```python
from build123d import *

# Parameters (mm, degrees)
RESSALTO_EXTRUS_O1_DEPTH = 1.5
ESBO_O2_R                = 0.1
RESSALTO_EXTRUS_O2_DEPTH = 0.1


with BuildPart() as part:
    # Esboço1 → Ressalto-extrusão1 (new body)
    with BuildSketch(Plane(origin=(0, 0, 0), x_dir=(1, 0, 0), z_dir=(0, 1, 0))):
        with BuildLine():
            Line((-3.97649343, 1.5), (-15, 1.5))
            ThreePointArc((-15, 1.5), (-16.358835062, 2.062847912), (-16.921682974, 3.421682974))
            Line((-16.921682974, 3.421682974), (-16.921682974, -3))
            ThreePointArc((-16.921682974, -3), (-16.482343146, -1.939339828), (-15.421682974, -1.5))
            Line((-15.421682974, -1.5), (-3.97649343, -1.5))
            ThreePointArc((-3.97649343, -1.5), (4.25, 0), (-3.97649343, 1.5))
        make_face()
    extrude(amount=RESSALTO_EXTRUS_O1_DEPTH)

    # Esboço2 → Ressalto-extrusão2 (add)
    with BuildSketch(Plane(origin=(0, 1.5, 0), x_dir=(1, 0, 0), z_dir=(0, 1, 0))):
        Circle(ESBO_O2_R)
    extrude(amount=RESSALTO_EXTRUS_O2_DEPTH)


solid = part.part
```
Build history of the part. All positions in model axes, mm. A direction names the side the tool comes from. Coordinates: 2 decimals unless noted, no trailing zeros. Order: outer loops, then holes, each group sorted by start corner. A loop starts at its lowest first (then second) coordinate and runs counter-clockwise, first axis right, second up. Notation, with made-up numbers: M 33,4 L 74,4 A20 ccw 74,38 Z; hole C -37.75,89 d2. An arc over 180 degrees is marked long. One line per question, with ' | ' between items. Start each with the question number.
1. Tool access for faces 4 (the face through (-16.494, 0.74, 1.951)), 5 (the face through (-9, 1, -1.5)), 6 (the face through (4.247, 0.74, 0.165)): list every direction of +Z, -Z, +X, -X, +Y, -Y with a clear straight run to the whole face (end or side of a thin tool).
2. Cut at C-C (x = -8.5). Write the cut outline in (y, z), plus the area to 3 significant figures.
3. Cut at B-B (z = 2.25). Write the cut outline in (x, y).
4. Cut at A-A (y = 0.85). Write the cut outline in (x, z).
5. Mould opens along X. For faces 1 (the face through (-4, 1.5, 0)), 2 (the face through (-16.344, 0.74, -2.048)), 3 (the face through (-16.922, 1, 0)) say: +X half, -X half, draft (parallel to the pull), parting line (faces both ways), or undercut.
6. Cut at D-D (z = 3.5). Write the cut outline in (x, y).
7. Flat gauge pins, fed straight in: P1, Ø0.8, axis at x = -7, y = 1, coming from the -Z side; P2, Ø2, axis at x = -0.5, z = -1.5, coming from the -Y side; P3, Ø2.5, axis at x = -3, z = 0, coming from the +Y side. Where does each tip first touch, or does it go through?
8. Wall check: line 1 along Z through (x, y) = (-12.5, 0.75); line 2 along X through (y, z) = (0.9, 2); line 3 along Y through (x, z) = (1, -2). Give the ranges that are in metal, low to high. Write a range as [from, to].
The answers:
1) face 4: +Z, +Y, -Y | face 5: -Z, +Y, -Y | face 6: +Y, -Y
2) outline: M 0,-1.5 L 1.5,-1.5 L 1.5,1.5 L 0,1.5 Z | area: 4.50 mm2
3) outline: M -16.92,0 L -16.72,0 L -16.72,1.5 L -16.92,1.5 Z; M -3.61,0 L 3.61,0 L 3.61,1.5 L -3.61,1.5 Z
4) outline: M -16.92,-3.42 A1.92 cw -15,-1.5 L -3.98,-1.5 A4.25 ccw long -3.98,1.5 L -15.42,1.5 A1.5 cw -16.92,3 Z
5) face 1: draft | face 2: undercut | face 3: -X half
6) outline: M -2.41,0 L 2.41,0 L 2.41,1.5 L -2.41,1.5 Z
7) P1: stops at z = -1.5 | P2: stops at y = 0 | P3: stops at y = 1.5
8) line 1: z = [-1.5, 1.5] | line 2: x = [-16.92, -16.54], [-3.75, 3.75] | line 3: y = [0, 1.5]
